from build123d import *

# Parameters (mm, degrees)
BOSS_EXTRUDE1_DEPTH      = 20.32
SKETCH2_W                = 58.42
SKETCH2_H                = 52.07
BOSS_EXTRUDE2_DEPTH      = 3.81
SKETCH3_W                = 12.7
SKETCH3_H                = 20.32
CUT_EXTRUDE1_DEPTH       = 3.81
FILLET2_R                = 2.54
SKETCH4_W                = 10.16
SKETCH4_H                = 5.08
BOSS_EXTRUDE3_DEPTH      = 10.16
CHAMFER1_SIZE            = 0.762
SKETCH5_W                = 10.16
SKETCH5_H                = 5.08
BOSS_EXTRUDE4_DEPTH      = 10.16
CHAMFER2_SIZE            = 0.762
CHAMFER2_OF_MIRROR1_SIZE = 0.762
M3_CLEARANCE_HOLE1_D     = 3.4
M3_CLEARANCE_HOLE2_D     = 3.4
CUT_EXTRUDE2_REACH       = 61.966
SKETCH13_W               = 44.45
SKETCH13_H               = 16.51
SKETCH15_W               = 13.462
SKETCH15_H               = 7.366
CUT_EXTRUDE4_DEPTH       = 79.475827011
FILLET3_R                = 2.54
SKETCH16_W               = 6.35
SKETCH16_H               = 3.81
BOSS_EXTRUDE5_DEPTH      = 3.81
CHAMFER3_SIZE            = 0.762
M3_CLEARANCE_HOLE4_D     = 3.4
CUT_EXTRUDE5_DEPTH       = 3.302
FILLET4_R                = 2.54


with BuildPart() as part:
    # Sketch1 → Boss-Extrude1 (new body)
    with BuildSketch(Plane(origin=(0, 0, 0), x_dir=(1, 0, 0), z_dir=(0, 1, 0))):
        Polygon((-27.305, 22.225), (-27.305, 26.035), (31.115, 26.035), (31.115, -26.035), (-27.305, -26.035), (-27.305, -22.225), (27.305, -22.225), (27.305, 22.225), align=None)
    extrude(amount=BOSS_EXTRUDE1_DEPTH)

    # Sketch2 → Boss-Extrude2 (add)
    with BuildSketch(Plane(origin=(0, 20.32, 0), x_dir=(1, 0, 0), z_dir=(0, 1, 0))):
        with Locations((1.905, 0)):
            Rectangle(SKETCH2_W, SKETCH2_H)
    extrude(amount=BOSS_EXTRUDE2_DEPTH)

    # Sketch3 → Cut-Extrude1 (cut)
    with BuildSketch(Plane.ZY.offset(-27.305)):
        with Locations((-15.875, 10.16)):
            Rectangle(SKETCH3_W, SKETCH3_H)
        with Locations((15.875, 10.16)):
            Rectangle(SKETCH3_W, SKETCH3_H)
    extrude(amount=-CUT_EXTRUDE1_DEPTH, mode=Mode.SUBTRACT)

    # Fillet2
    fillet2_edges = [part.edges().sort_by_distance(p)[0] for p in [
        (31.115, 12.065, -26.035),
        (31.115, 12.065, 26.035),
        (31.115, 24.13, 0),
    ]]
    fillet(fillet2_edges, radius=FILLET2_R)

    # Sketch4 → Boss-Extrude3 (add)
    with BuildSketch(Plane(origin=(31.115, 0, 0), x_dir=(0, 0, -1), z_dir=(1, 0, 0))):
        with Locations((0, 2.54)):
            Rectangle(SKETCH4_W, SKETCH4_H)
    extrude(amount=BOSS_EXTRUDE3_DEPTH)

    # Chamfer1
    chamfer1_edges = [part.edges().sort_by_distance(p)[0] for p in [
        (31.115, 2.54, 5.08),
        (36.195, 5.08, 5.08),
        (31.115, 2.54, -5.08),
        (31.115, 5.08, 0),
        (36.195, 5.08, -5.08),
        (41.275, 2.54, 5.08),
        (41.275, 2.54, -5.08),
        (41.275, 5.08, 0),
    ]]
    chamfer(chamfer1_edges, length=CHAMFER1_SIZE)

    # Sketch5 → Boss-Extrude4 (add)
    with BuildSketch(Plane.XY.offset(26.035)):
        with Locations((-14.605, 2.54)):
            Rectangle(SKETCH5_W, SKETCH5_H)
    boss_extrude4 = extrude(amount=BOSS_EXTRUDE4_DEPTH)

    # Chamfer2
    chamfer2_edges = [part.edges().sort_by_distance(p)[0] for p in [
        (-19.685, 2.54, 26.035),
        (-19.685, 5.08, 31.115),
        (-9.525, 2.54, 26.035),
        (-14.605, 5.08, 26.035),
        (-9.525, 5.08, 31.115),
        (-19.685, 2.54, 36.195),
        (-9.525, 2.54, 36.195),
        (-14.605, 5.08, 36.195),
    ]]
    chamfer(chamfer2_edges, length=CHAMFER2_SIZE)

    # Mirror1: Boss-Extrude4 across plane
    add(boss_extrude4.mirror(Plane.XY))

    # Chamfer2 of Mirror1
    chamfer2_of_mirror1_edges = [part.edges().sort_by_distance(p)[0] for p in [
        (-19.685, 2.54, -26.035),
        (-19.685, 5.08, -31.115),
        (-9.525, 2.54, -26.035),
        (-14.605, 5.08, -26.035),
        (-9.525, 5.08, -31.115),
        (-19.685, 2.54, -36.195),
        (-9.525, 2.54, -36.195),
        (-14.605, 5.08, -36.195),
    ]]
    chamfer(chamfer2_of_mirror1_edges, length=CHAMFER2_OF_MIRROR1_SIZE)

    # M3 Clearance Hole1 (through all)
    with Locations(Plane(origin=(0, 5.08, 0), x_dir=(1, 0, 0), z_dir=(0, 1, 0))):
        with Locations((-14.605, -31.115)):
            m3_clearance_hole1 = Hole(M3_CLEARANCE_HOLE1_D / 2)

    # Mirror2: M3 Clearance Hole1 across plane
    add(m3_clearance_hole1.mirror(Plane.XY), mode=Mode.SUBTRACT)

    # M3 Clearance Hole2 (through all)
    with Locations(Plane(origin=(0, 5.08, 0), x_dir=(1, 0, 0), z_dir=(0, 1, 0))):
        with Locations((36.195, 0)):
            Hole(M3_CLEARANCE_HOLE2_D / 2)

    # Sketch13 → Cut-Extrude2 (cut, up to next)
    with BuildSketch(Plane(origin=(0, 24.13, 0), x_dir=(1, 0, 0), z_dir=(0, 1, 0)), mode=Mode.PRIVATE) as cut_extrude2_sk1:
        with Locations((0, -10.795)):
            Rectangle(SKETCH13_W, SKETCH13_H)
    cut_extrude2_tool1 = extrude(cut_extrude2_sk1.sketch, amount=-CUT_EXTRUDE2_REACH, mode=Mode.PRIVATE) & part.part
    # Sketch13 → Cut-Extrude2 (cut, up to next)
    with BuildSketch(Plane(origin=(0, 24.13, 0), x_dir=(1, 0, 0), z_dir=(0, 1, 0)), mode=Mode.PRIVATE) as cut_extrude2_sk2:
        with Locations((0, 10.795)):
            Rectangle(SKETCH13_W, SKETCH13_H)
    cut_extrude2_tool2 = extrude(cut_extrude2_sk2.sketch, amount=-CUT_EXTRUDE2_REACH, mode=Mode.PRIVATE) & part.part
    add(cut_extrude2_tool1.solids().sort_by_distance((0, 24.13, 10.795))[0], mode=Mode.SUBTRACT)
    add(cut_extrude2_tool2.solids().sort_by_distance((0, 24.13, -10.795))[0], mode=Mode.SUBTRACT)

    # Sketch15 → Cut-Extrude4 (cut, through all)
    with BuildSketch(Plane(origin=(0, 0, -26.035), x_dir=(-1, 0, 0), z_dir=(0, 0, -1))):
        Polygon((-22.225, 0), (4.953, 0), (4.953, 9.652), (4.953, 17.018), (-22.225, 17.018), align=None)
        with Locations((15.494, 13.335)):
            Rectangle(SKETCH15_W, SKETCH15_H)
    extrude(amount=-CUT_EXTRUDE4_DEPTH, mode=Mode.SUBTRACT)

    # Fillet3
    fillet3_edges = [part.edges().sort_by_distance(p)[0] for p in [
        (-22.225, 22.225, 19.05),
        (-22.225, 22.225, 2.54),
        (1.905, 20.32, -22.225),
        (22.225, 22.225, 2.54),
        (22.225, 22.225, 19.05),
        (22.225, 22.225, -19.05),
        (22.225, 22.225, -2.54),
        (-22.225, 22.225, -2.54),
        (-22.225, 22.225, -19.05),
        (22.225, 17.018, 24.13),
        (22.225, 17.018, -24.13),
        (-4.953, 17.018, 24.13),
        (-4.953, 17.018, -24.13),
        (-22.225, 17.018, 24.13),
        (-22.225, 17.018, -24.13),
        (-22.225, 9.652, 24.13),
        (-22.225, 9.652, -24.13),
        (-8.763, 9.652, 24.13),
        (-8.763, 9.652, -24.13),
        (-8.763, 17.018, 24.13),
        (-8.763, 17.018, -24.13),
        (29.21, 20.32, -9.525),
        (29.21, 20.32, 9.525),
        (1.905, 20.32, 22.225),
    ]]
    fillet(fillet3_edges, radius=FILLET3_R)

    # Sketch16 → Boss-Extrude5 (add)
    with BuildSketch(Plane(origin=(0, 24.13, 0), x_dir=(1, 0, 0), z_dir=(0, 1, 0))):
        with Locations((-27.305, 0)):
            Rectangle(SKETCH16_W, SKETCH16_H)
    extrude(amount=-BOSS_EXTRUDE5_DEPTH)

    # Chamfer3
    chamfer3_edges = [part.edges().sort_by_distance(p)[0] for p in [
        (-28.8925, 20.32, -1.905),
        (-28.8925, 20.32, 1.905),
        (-30.48, 20.32, 0),
        (-30.48, 22.225, -1.905),
        (-30.48, 22.225, 1.905),
    ]]
    chamfer(chamfer3_edges, length=CHAMFER3_SIZE)

    # M3 Clearance Hole4 (through all)
    with Locations(Plane(origin=(0, 24.13, 0), x_dir=(1, 0, 0), z_dir=(0, 1, 0))):
        with Locations((25.286866606, -21.9964), (25.286866606, 21.9964)):
            Hole(M3_CLEARANCE_HOLE4_D / 2)

    # Sketch22 → Cut-Extrude5 (cut)
    with BuildSketch(Plane.XZ.offset(-20.32)):
        Polygon((28.953040816, 21.9964), (27.119953711, 25.1714), (23.453779502, 25.1714), (21.620692397, 21.9964), (23.453779502, 18.8214), (27.119953711, 18.8214), align=None)
        Polygon((28.953040816, -21.9964), (27.119953711, -18.8214), (23.453779502, -18.8214), (21.620692397, -21.9964), (23.453779502, -25.1714), (27.119953711, -25.1714), align=None)
    extrude(amount=CUT_EXTRUDE5_DEPTH, mode=Mode.SUBTRACT)

    # Fillet4
    # the kernel refuses this fillet: 2.54 mm, written as the material it takes off along each edge
    with BuildSketch(Plane(origin=(28.575, 21.59, 23.495), x_dir=(0, 0, 1), z_dir=(0, 1, 0))) as fillet4_piece_1_section:
        Polygon((0, 0), (FILLET4_R, 0), (FILLET4_R, FILLET4_R), (0, FILLET4_R), align=None)
    fillet4_piece_1 = extrude(amount=FILLET4_R, mode=Mode.PRIVATE)
    fillet4_piece_1 = fillet4_piece_1 - Plane(origin=(28.575, 21.59, 23.495), x_dir=(-0.7071067811865475, 0, -0.7071067811865475), z_dir=(0, 1, 0)) * Sphere(FILLET4_R, mode=Mode.PRIVATE)
    add(fillet4_piece_1, mode=Mode.SUBTRACT)
    with BuildSketch(Plane(origin=(28.575, 21.59, -23.495), x_dir=(0, 0, -1), z_dir=(0, 1, 0))) as fillet4_piece_2_section:
        Polygon((0, 0), (FILLET4_R, 0), (FILLET4_R, -FILLET4_R), (0, -FILLET4_R), align=None)
    fillet4_piece_2 = extrude(amount=FILLET4_R, mode=Mode.PRIVATE)
    fillet4_piece_2 = fillet4_piece_2 - Plane(origin=(28.575, 21.59, -23.495), x_dir=(-0.7071067811865475, 0, 0.7071067811865475), z_dir=(0, 1, 0)) * Sphere(FILLET4_R, mode=Mode.PRIVATE)
    add(fillet4_piece_2, mode=Mode.SUBTRACT)
    with BuildSketch(Plane(origin=(28.575, 24.13, 26.035), x_dir=(0, 0, -1), z_dir=(-1, 0, 0)), Plane(origin=(-33.655, 24.13, -26.035), x_dir=(0, 0, 1), z_dir=(1, 0, 0))) as fillet4_piece_3:
        with BuildLine():
            CenterArc((FILLET4_R, FILLET4_R), FILLET4_R, 180, 90)
            Line((0, FILLET4_R), (0, 0))
            Line((0, 0), (FILLET4_R, 0))
        make_face()
    extrude(amount=62.23, mode=Mode.SUBTRACT)


solid = part.part
Could you check a few things on this model? Use its own coordinates, in mm. A direction names the side the tool comes from. Round coordinates to 2 decimals unless told otherwise and drop trailing zeros. Loops run counter-clockwise (first coordinate to the right, second up) from the corner with the lowest first, then second, coordinate; pieces in that order, holes last. Notation, with made-up numbers: (39.25, 0) - (63.25, 0) arc R25 cw to (63.25, 34) - close; hole circle Ø3 at (25.5, -7.5). An arc over 180 degrees is marked (long way). Write item = value, one per line.
1) Imagine slicing it at A-A (x = 0). Please give me the cut outline in (y, z) (3 decimals).
Computed:
outline = (17.018, -26.035) - (21.59, -26.035) arc R2.54 ccw to (24.13, -23.495) - (24.13, -19.05) - (20.32, -19.05) - (20.32, -19.685) arc R2.54 cw to (17.78, -22.225) - (17.018, -22.225) - close; (17.018, 22.225) - (17.78, 22.225) arc R2.54 cw to (20.32, 19.685) - (20.32, 19.05) - (24.13, 19.05) - (24.13, 23.495) arc R2.54 ccw to (21.59, 26.035) - (17.018, 26.035) - close; (20.32, -2.54) - (24.13, -2.54) - (24.13, 2.54) - (20.32, 2.54) - close
2) I need wall thicknesses on line 1 along Z through (x, y) = (28.5, 7.25) (3 decimals); line 2 along Z through (x, y) = (9.5, 21.25) (3 decimals); line 3 along Y through (x, z) = (37, -2). Which ranges of each line are inside material? Lowest first, please. Write a range as from..to.
Computed:
line_1 = -26.035..-22.225, -9.525..9.525, 22.225..26.035
line_2 = -26.035..-19.05, -2.54..2.54, 19.05..26.035
line_3 = 0..5.08
3) Imagine slicing it at C-C (z = 14). Please give me the cut outline in (x, y) (3 decimals).
Computed:
outline = (-27.305, 20.32) - (-22.225, 20.32) - (-22.225, 24.13) - (-27.305, 24.13) - close; (22.225, 20.32) - (31.115, 20.32) - (31.115, 21.59) arc R2.54 ccw to (28.575, 24.13) - (22.225, 24.13) - close
4) Imagine slicing it at B-B (z = 0). Please give me the cut outline in (x, y) (3 decimals), and give its area (3 significant figures).
Computed:
outline = (-30.48, 21.082) - (-29.718, 20.32) - (27.305, 20.32) - (27.305, 0) - (34.495, 0) - (34.495, 5.08) - (31.877, 5.08) - (31.115, 5.842) - (31.115, 21.59) arc R2.54 ccw to (28.575, 24.13) - (-30.48, 24.13) - close; (37.895, 0) - (41.275, 0) - (41.275, 4.318) - (40.513, 5.08) - (37.895, 5.08) - close
area = 345 mm2
5) If we mould it in two halves opening along X, with no side actions, what happens to faces 4 (the flat face through (-29, 23, -1.905)), 5 (the flat face through (-30.48, 23, 0)), 6 (the cylindrical face through (21.501, 22.198, -18.286))? For each: pulls with the +X half, pulls with the -X half, needs draft (parallel to the pull), parting line crosses it, or undercut.
Computed:
face_4 = needs draft
face_5 = pulls with the -X half
face_6 = undercut
6) On a 3-axis mill with a long thin cutter (end or side, diameter ignored), from which of +Z, -Z, +X, -X, +Y, -Y can I reach the whole of each face in a straight line? I mean faces 1 (the cylindrical face through (29.731, 19.556, -21.501)), 2 (the cylindrical face through (-9.527, 10.376, -24.103)), 3 (the flat face through (-9.525, 2, 31)). Say none if no direction works.
Computed:
face_1 = +X, -X, -Y
face_2 = +Z, -Z
face_3 = +Z, +X, +Y, -Y
7) I'm going to push flat-ended pins straight in: P1, Ø4.5, axis at x = 36.5, y = 1.5, coming from the +Z side; P2, Ø3, axis at x = 29, y = 12.5, coming from the -Z side (3 decimals); P3, Ø6, axis at x = -7.5, y = 17.5, coming from the +Z side (3 decimals); P4, Ø4.5, axis at x = 25.29, z = -22, coming from the -Y side. Where does each tip first touch, or does it pass through?
Computed:
P1 = 5.08
P2 = -26.035
P3 = 26.035
P4 = 0
